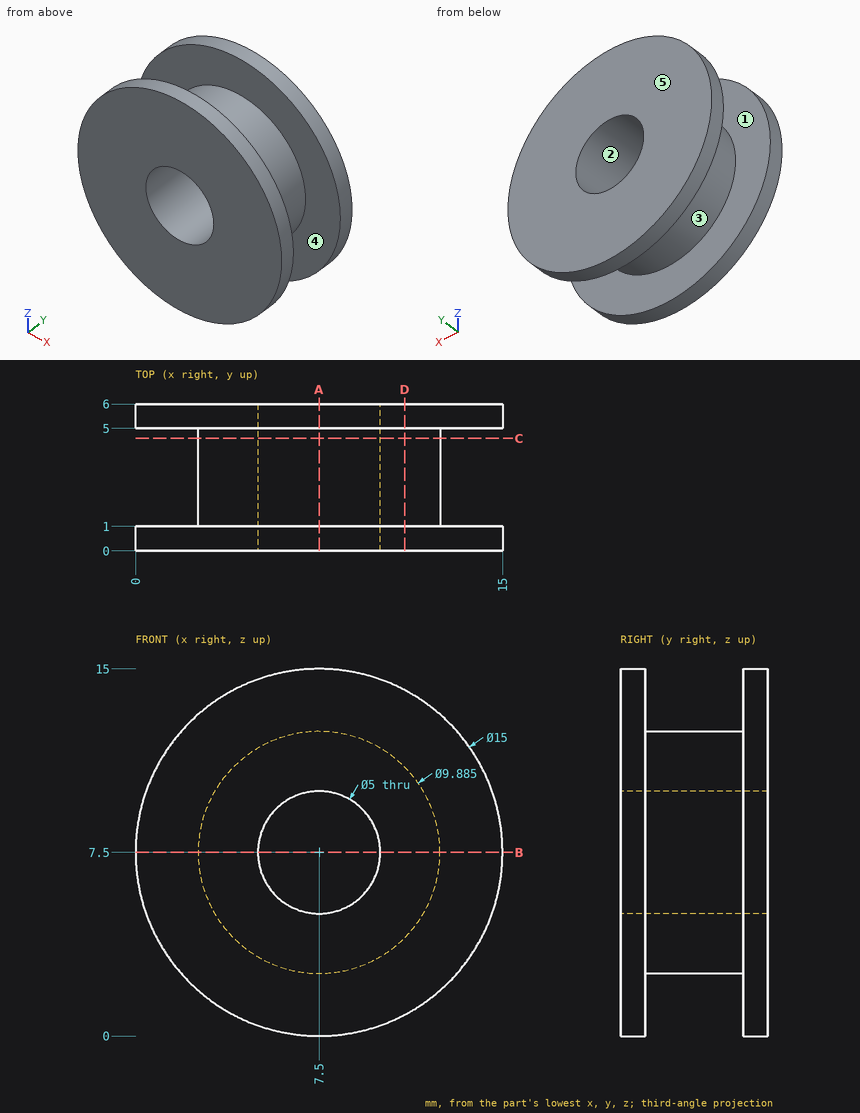
Study the drawing (mm; zero at the part's minimum x, y, z) and answer. A direction names the side the tool comes from. Coordinates: 2 decimals unless noted, no trailing zeros. Write each loop counter-clockwise with the first axis right and the second up, starting at its lowest first coordinate (ties: lowest second). Pieces come first, ordered by that corner, then holes.
Q1. A cutting plane is placed at B-B, the plane z = 7.5. Give the vertices of the cut face in (x, y).
Q2. A cutting plane is placed at D-D, the plane x = 11. Give the vertices of the cut face in (y, z).
Q3. Determine the mould class of the marked faces 1, 2 and 3 for opening direction X: released by +X, released by -X, zero draft, split by the parting line, or undercut.
Q4. Each of these flat-tipped pins is pushed along its axis until it touches: pin 1 Ø3 at (x, y) = (4, 4) entering from +Z; pin 2 Ø3 at (x, z) = (7.5, 7.5) entering from +Y; pin 3 Ø1.5 at (y, z) = (5, 12.5) entering from -X. Where does it stop, or does it pass through?
Q5. Which of the six approach directions +Z, -Z, +X, -X, +Y, -Y give full straight-line access (tool end or side, diameter ignored) to the marked faces 4 and 5?
Q6. A cutting plane is placed at C-C, the plane y = 4.6. Give the vertices of the cut face in (x, z) (1 decimal), then the cut area to 3 significant figures.
Q7. Find the intervals of material crossed by line 1 (Y direction, x = 13.5, z = 6.5); line 2 (Z direction, x = 7.5, y = 4.7); line 3 (Z direction, x = 7.75, y = 5.25), in increasing order.
Q8. A cutting plane is placed at A-A, the plane x = 7.5. Give the vertices of the cut face in (y, z), then the cut area to 3 significant figures.
Findings below:
1. outline: (0, 0) - (5, 0) - (5, 6) - (0, 6) - (0, 5) - (2.56, 5) - (2.56, 1) - (0, 1) - close; (10, 0) - (15, 0) - (15, 1) - (12.44, 1) - (12.44, 5) - (15, 5) - (15, 6) - (10, 6) - close
2. outline: (0, 0.87) - (1, 0.87) - (1, 4.01) - (5, 4.01) - (5, 0.87) - (6, 0.87) - (6, 14.13) - (5, 14.13) - (5, 10.99) - (1, 10.99) - (1, 14.13) - (0, 14.13) - close
3. face 1: zero draft
3. face 2: undercut
3. face 3: split by the parting line
4. pin 1: stops at z = 14.61
4. pin 2: passes through
4. pin 3: stops at x = 1.32
5. face 4: none
5. face 5: +Z, -Z, +X, -X, +Y
6. outline: circle Ø9.9 at (7.5, 7.5); hole circle Ø5 at (7.5, 7.5)
6. area: 57.1 mm2
7. line 1: y = 0 to 1, 5 to 6
7. line 2: z = 2.56 to 5, 10 to 12.44
7. line 3: z = 0 to 5.01, 9.99 to 15
8. outline: (0, 0) - (1, 0) - (1, 2.56) - (5, 2.56) - (5, 0) - (6, 0) - (6, 5) - (0, 5) - close; (0, 10) - (6, 10) - (6, 15) - (5, 15) - (5, 12.44) - (1, 12.44) - (1, 15) - (0, 15) - close
8. area: 39.5 mm2
